Geometry: final body of the model. Coordinates: model frame, mm. A direction names the side the tool comes from. Round coordinates to 2 decimals unless told otherwise and drop trailing zeros. Write each loop counter-clockwise with the first axis right and the second up, starting at its lowest first coordinate (ties: lowest second). Pieces come first, ordered by that corner, then holes.
from build123d import *

# Parameters (mm, degrees)
BOSS_EXTRUDE1_DEPTH = 8
SKETCH2_R           = 30
BOSS_EXTRUDE2_DEPTH = 22
SKETCH3_R           = 3.8
CUT_EXTRUDE1_DEPTH  = 5
SKETCH4_R           = 3.8
CUT_EXTRUDE2_DEPTH  = 5


with BuildPart() as part:
    # Sketch1 → Boss-Extrude1 (new body)
    with BuildSketch(Plane.XY):
        with BuildLine():
            Line((-8.2, 39.150478924), (-8.2, 30.41397705))
            ThreePointArc((-8.2, 30.41397705), (-22.273863607, 22.273863607), (-30.41397705, 8.2))
            Line((-30.41397705, 8.2), (-39.150478924, 8.2))
            ThreePointArc((-39.150478924, 8.2), (-40, 0), (-39.150478924, -8.2))
            Line((-39.150478924, -8.2), (-30.41397705, -8.2))
            ThreePointArc((-30.41397705, -8.2), (-22.273863607, -22.273863607), (-8.2, -30.41397705))
            Line((-8.2, -30.41397705), (-8.2, -39.150478924))
            ThreePointArc((-8.2, -39.150478924), (0, -40), (8.2, -39.150478924))
            Line((8.2, -39.150478924), (8.2, -30.41397705))
            ThreePointArc((8.2, -30.41397705), (22.273863607, -22.273863607), (30.41397705, -8.2))
            Line((30.41397705, -8.2), (39.150478924, -8.2))
            ThreePointArc((39.150478924, -8.2), (40, 0), (39.150478924, 8.2))
            Line((39.150478924, 8.2), (30.41397705, 8.2))
            ThreePointArc((30.41397705, 8.2), (22.273863607, 22.273863607), (8.2, 30.41397705))
            Line((8.2, 30.41397705), (8.2, 39.150478924))
            ThreePointArc((8.2, 39.150478924), (0, 40), (-8.2, 39.150478924))
        make_face()
    extrude(amount=BOSS_EXTRUDE1_DEPTH)

    # Sketch2 → Boss-Extrude2 (add)
    with BuildSketch(Plane.XY.offset(8)):
        Circle(SKETCH2_R)
    extrude(amount=BOSS_EXTRUDE2_DEPTH)

    # Sketch3 → Cut-Extrude1 (cut)
    with BuildSketch(Plane.XY.offset(8)):
        with Locations((0, 35)):
            Circle(SKETCH3_R)
        with Locations((35, 0)):
            Circle(SKETCH3_R)
        with Locations((0, -35)):
            Circle(SKETCH3_R)
        with Locations((-35, 0)):
            Circle(SKETCH3_R)
    extrude(amount=-CUT_EXTRUDE1_DEPTH, mode=Mode.SUBTRACT)

    # Sketch4 → Cut-Extrude2 (cut)
    with BuildSketch(Plane.XY.offset(30)):
        with Locations((0, 22.5)):
            Circle(SKETCH4_R)
        with Locations((22.5, 0)):
            Circle(SKETCH4_R)
        with Locations((0, -22.5)):
            Circle(SKETCH4_R)
        with Locations((-22.5, 0)):
            Circle(SKETCH4_R)
    extrude(amount=-CUT_EXTRUDE2_DEPTH, mode=Mode.SUBTRACT)


solid = part.part
1) Section B-B on z = 27.25. Output: boundary loops of the cut face in (x, y), plus the area to 3 significant figures.
2) Reachability of faces 4 (the cylindrical face through (0, -40, 4)), 5 (the flat face through (35, 8.2, 4)), 6 (the flat face through (0, 23, 25)) from +Z, -Z, +X, -X, +Y, -Y: full face, straight path, thin tool, end or side. Return the list, or none.
3) Section A-A on y = 0. Output: boundary loops of the cut face in (x, z), plus the area to 3 significant figures.
4) Line query: probe 1 along Y at (x, z) = (0, 26.1); probe 2 along X at (y, z) = (3, 7); probe 3 along Y at (x, z) = (-35, 4.65). Output: solid intervals per line, ascending.
5) First-contact query: P1, Ø8.5, axis at x = -35.5, y = 0.5, coming from the +Z side; P2, Ø6, axis at x = -23.5, y = -1, coming from the +Z side; P3, Ø10, axis at y = -1, z = 19, coming from the -X side; P4, Ø1.5, axis at y = -20, z = 10, coming from the +X side. Flat tips, straight axial feed; report the tip coordinate or a pass-through.
6) Draft query along X for faces 1 (the flat face through (6, 30, 8)), 2 (the cylindrical face through (-2.8, 25.07, 27.54)), 3 (the flat face through (-8.2, 35, 4)). Return one class per face: pulls with the +X half, pulls with the -X half, needs draft (parallel to the pull), parting line crosses it, or undercut.
7) Section C-C on x = -35. Output: boundary loops of the cut face in (y, z), plus the area to 3 significant figures.
Filled in:
1. outline: circle Ø60 at (0, 0); hole circle Ø7.6 at (-22.5, 0); hole circle Ø7.6 at (0, -22.5); hole circle Ø7.6 at (0, 22.5); hole circle Ø7.6 at (22.5, 0)
1. area: 2,650 mm2
2. face 4: +Z, -Z, -Y
2. face 5: +Z, -Z, +X, +Y
2. face 6: +Z
3. outline: (-40, 0) - (40, 0) - (40, 8) - (38.8, 8) - (38.8, 3) - (31.2, 3) - (31.2, 8) - (30, 8) - (30, 30) - (26.3, 30) - (26.3, 25) - (18.7, 25) - (18.7, 30) - (-18.7, 30) - (-18.7, 25) - (-26.3, 25) - (-26.3, 30) - (-30, 30) - (-30, 8) - (-31.2, 8) - (-31.2, 3) - (-38.8, 3) - (-38.8, 8) - (-40, 8) - close
3. area: 1,810 mm2
4. probe 1: y = -30 to -26.3, -18.7 to 18.7, 26.3 to 30
4. probe 2: x = -39.89 to -37.33, -32.67 to 32.67, 37.33 to 39.89
4. probe 3: y = -8.2 to -3.8, 3.8 to 8.2
5. P1: stops at z = 8
5. P2: stops at z = 30
5. P3: stops at x = -30
5. P4: stops at x = 23.01
6. face 1: needs draft
6. face 2: undercut
6. face 3: pulls with the -X half
7. outline: (-8.2, 0) - (8.2, 0) - (8.2, 8) - (3.8, 8) - (3.8, 3) - (-3.8, 3) - (-3.8, 8) - (-8.2, 8) - close
7. area: 93.2 mm2
